The model under review builds one solid part; all positions refer to its coordinate system, in mm. A direction names the side the tool comes from. Coordinates: 2 decimals unless noted, no trailing zeros. Order: outer loops, then holes, each group sorted by start corner. A loop starts at its lowest first (then second) coordinate and runs counter-clockwise, first axis right, second up.
```python
from build123d import *

# Parameters (mm, degrees)
SKETCH1_R                = 36.8
SKETCH1_R_2              = 35.2
BOSS_EXTRUDE1_DEPTH      = 100
BOSS_EXTRUDE2_DEPTH      = 10
BOSS_EXTRUDE2_DEPTH_BACK = 5
SKETCH2_R                = 38.3
SKETCH2_R_2              = 36.8
CHAMFER1_SIZE            = 1.5
BOSS_EXTRUDE3_START      = 30
BOSS_EXTRUDE3_DEPTH      = 30
SKETCH7_R                = 1.75
CUT_EXTRUDE1_DEPTH       = 116.043019012
CUT_EXTRUDE2_REACH       = 153.112
CUT_EXTRUDE3_REACH       = 138.3
CUT_EXTRUDE3_END_RADIUS  = 35.2
SKETCH9_R                = 5


with BuildPart() as part:
    # Sketch1 → Boss-Extrude1 (new body)
    with BuildSketch(Plane.XY):
        Circle(SKETCH1_R)
        Circle(SKETCH1_R_2, mode=Mode.SUBTRACT)
    extrude(amount=BOSS_EXTRUDE1_DEPTH)

    # Sketch2 → Boss-Extrude2 (add, two sides: drawn at the far end of the back side and taken through both)
    with BuildSketch(Plane(origin=(0, 0, 0), x_dir=(-1, 0, 0), z_dir=(0, 0, -1)).offset(-BOSS_EXTRUDE2_DEPTH_BACK)):
        Circle(SKETCH2_R)
        Circle(SKETCH2_R_2, mode=Mode.SUBTRACT)
    extrude(amount=BOSS_EXTRUDE2_DEPTH + BOSS_EXTRUDE2_DEPTH_BACK)

    # Chamfer1
    chamfer1_edges = [part.edges().sort_by_distance(p)[0] for p in [
        (-36.8, 0, 5),
    ]]
    chamfer(chamfer1_edges, length=CHAMFER1_SIZE - 0.0001)  # a hair under: the kernel refuses the full size

    # Sketch6 → Boss-Extrude3 (add)
    with BuildSketch(Plane(origin=(0, 0, -10), x_dir=(-1, 0, 0), z_dir=(0, 0, -1)).offset(BOSS_EXTRUDE3_START)):
        with BuildLine():
            Line((-31.046363436, 22.427958387), (-32.43120853, 23.227499075))
            Line((-32.43120853, 23.227499075), (-35.462297443, 24.977499075))
            Line((-35.462297443, 24.977499075), (-38.147666087, 26.527897384))
            Line((-38.147666087, 26.527897384), (-39.147666087, 24.795846576))
            Line((-39.147666087, 24.795846576), (-36.462297443, 23.245448267))
            Line((-36.462297443, 23.245448267), (-33.43120853, 21.495448267))
            Line((-33.43120853, 21.495448267), (-32.177933832, 20.771869783))
            Line((-32.177933832, 20.771869783), (-30.861043972, 20.045846576))
            ThreePointArc((-30.861043972, 20.045846576), (18.4, 31.869734859), (32.790734361, -16.703524779))
            Line((32.790734361, -16.703524779), (34.077933832, -17.480973249))
            Line((34.077933832, -17.480973249), (35.33120853, -18.204551733))
            Line((35.33120853, -18.204551733), (38.362297443, -19.954551733))
            Line((38.362297443, -19.954551733), (41.047666087, -21.504950042))
            Line((41.047666087, -21.504950042), (42.047666087, -19.772899234))
            Line((42.047666087, -19.772899234), (39.362297443, -18.222500925))
            Line((39.362297443, -18.222500925), (36.33120853, -16.472500925))
            Line((36.33120853, -16.472500925), (34.946363436, -15.672960237))
            ThreePointArc((34.946363436, -15.672960237), (19.15, 33.168772965), (-31.046363436, 22.427958387))
        make_face()
        with BuildLine():
            Line((-34.946363436, 15.672960237), (-36.33120853, 16.472500925))
            Line((-36.33120853, 16.472500925), (-39.362297443, 18.222500925))
            Line((-39.362297443, 18.222500925), (-42.047666087, 19.772899234))
            Line((-42.047666087, 19.772899234), (-41.047666087, 21.504950042))
            Line((-41.047666087, 21.504950042), (-38.362297443, 19.954551733))
            Line((-38.362297443, 19.954551733), (-35.33120853, 18.204551733))
            Line((-35.33120853, 18.204551733), (-34.077933832, 17.480973249))
            Line((-34.077933832, 17.480973249), (-32.743288904, 16.796339832))
            ThreePointArc((-32.743288904, 16.796339832), (-18.4, -31.869734859), (30.917701437, -19.958350079))
            Line((30.917701437, -19.958350079), (32.177933832, -20.771869783))
            Line((32.177933832, -20.771869783), (33.43120853, -21.495448267))
            Line((33.43120853, -21.495448267), (36.462297443, -23.245448267))
            Line((36.462297443, -23.245448267), (39.147666087, -24.795846576))
            Line((39.147666087, -24.795846576), (38.147666087, -26.527897384))
            Line((38.147666087, -26.527897384), (35.462297443, -24.977499075))
            Line((35.462297443, -24.977499075), (32.43120853, -23.227499075))
            Line((32.43120853, -23.227499075), (31.046363436, -22.427958387))
            ThreePointArc((31.046363436, -22.427958387), (-19.15, -33.168772965), (-34.946363436, 15.672960237))
        make_face()
    extrude(amount=-BOSS_EXTRUDE3_DEPTH)

    # Sketch7 → Cut-Extrude1 (cut, symmetric)
    with BuildSketch(Plane(origin=(0, 0, 0), x_dir=(0, 0, 1), z_dir=(0.500000000000001, -0.866025403784438, 0))):
        with Locations(Location((-29.75, 41.45, 0), (0, 0, 270))):
            Circle(SKETCH7_R)
        with Locations(Location((-15.25, 41.45, 0), (0, 0, 270))):
            Circle(SKETCH7_R)
    cut_extrude1 = extrude(amount=CUT_EXTRUDE1_DEPTH, both=True, mode=Mode.SUBTRACT)

    # Mirror1: Cut-Extrude1 across plane
    add(cut_extrude1.mirror(Plane(origin=(0, 0, 0), x_dir=(0, 0, 1), z_dir=(0.866025403784438, 0.500000000000001, 0))), mode=Mode.SUBTRACT)

    # Cut-Extrude2: up to this face of the body (flat: up to its plane)
    cut_extrude2_end = Plane(part.part.faces().sort_by_distance((35.759138818, 0, 0))[0])
    # Sketch8 → Cut-Extrude2 (cut, up to the picked face)
    with BuildSketch(Plane(origin=(0, 0, -40), x_dir=(-1, 0, 0), z_dir=(0, 0, -1)), mode=Mode.PRIVATE) as cut_extrude2_sk1:
        with BuildLine():
            ThreePointArc((31.085732423, -20.066819373), (32.069109105, -18.454599459), (32.968944874, -16.794304805))
            ThreePointArc((32.968944874, -16.794304805), (18.5, 32.04293994), (-31.028767037, 20.154791395))
            ThreePointArc((-31.028767037, 20.154791395), (-32.016706501, 18.545363432), (-32.921241561, 16.887624287))
            ThreePointArc((-32.921241561, 16.887624287), (-18.5, -32.04293994), (31.085732423, -20.066819373))
        make_face()
    cut_extrude2_tool1 = split(extrude(cut_extrude2_sk1.sketch, amount=-CUT_EXTRUDE2_REACH, mode=Mode.PRIVATE), bisect_by=cut_extrude2_end, keep=Keep.BOTH, mode=Mode.PRIVATE)
    add(cut_extrude2_tool1.solids().sort_by(Axis((0, 0, -40), (0, 0, 1)))[0], mode=Mode.SUBTRACT)

    # Cut-Extrude3: up to this cylinder (the profile starts outside it)
    cut_extrude3_end = Plane(origin=(0, 0, 15), z_dir=(0, 0, -1)) * Cylinder(CUT_EXTRUDE3_END_RADIUS, 348, mode=Mode.PRIVATE)
    # Sketch9 → Cut-Extrude3 (cut, up to the surface)
    with BuildSketch(Plane(origin=(-18.4, 31.869734859, 0), x_dir=(0.8660254037844382, 0.500000000000001, 0), z_dir=(-0.500000000000001, 0.8660254037844382, 0)), mode=Mode.PRIVATE) as cut_extrude3_sk1:
        with Locations(Location((0, -15, 0), (0, 0, 180))):
            Circle(SKETCH9_R)
    cut_extrude3_tool1 = extrude(cut_extrude3_sk1.sketch, amount=-CUT_EXTRUDE3_REACH, mode=Mode.PRIVATE) - cut_extrude3_end
    add(cut_extrude3_tool1.solids().sort_by_distance((-18.4, 31.869735, 15))[0], mode=Mode.SUBTRACT)


solid = part.part
```
(1) Machinability: for faces 1 (the face through (-22, 31, -40)), 2 (the face through (38, 18, -10)), 3 (the face through (-38, -19, -10)), which of the approach directions +Z, -Z, +X, -X, +Y, -Y give a long, thin tool a straight path to every point of the face, cutting with its end or side? Answer none if there is none.
A:
face 1: -Z, +X, -X, +Y, -Y
face 2: +Z, +X, +Y
face 3: +Z, -X, -Y
(2) For pin 1 Ø6.5 at (x, y) = (-36, -24) entering from +Z; pin 2 Ø2.5 at (x, y) = (32, 18.5) entering from -Z; pin 3 Ø12 at (x, z) = (8.5, 30) entering from -Y (3 decimals); pin 4 Ø6 at (y, z) = (-21, -14.5) entering from -X, all flat-tipped, find the tip position at first contact; note any pin that passes through.
A:
pin 1: stops at z = -10
pin 2: stops at z = -10
pin 3: stops at y = -36.715
pin 4: stops at x = -42.05
(3) We need section C-C, the plane z = 23.5. Write out the cut boundary in (x, y).
A:
outline: circle Ø73.6 at (0, 0); hole circle Ø70.4 at (0, 0)
(4) We need section D-D, the plane y = 32. Count the separate pieces of the cut face and the enclosed holes in it, and give its area (3 significant figures).
A:
separate pieces: 3
enclosed holes: 0
area: 900 mm2
(5) Wall thickness on probe 1 along X at (y, z) = (0, -25.5); probe 2 along Y at (x, z) = (1, 82); probe 3 along Y at (x, z) = (31.5, -5): over which ranges is each line inside the solid? List them lowest first.
A:
probe 1: x = -38.3 to -37, 37 to 38.3
probe 2: y = -36.79 to -35.19, 35.19 to 36.79
probe 3: y = -21.79 to -19.41, 19.41 to 21.79
(6) Draft analysis for pull direction Z (two halves, no side actions). For faces 4 (the face through (-36.64, -17.82, -31.3)), 5 (the face through (-33, -19, -10)), 6 (the face through (35, 24, -10)), state which applies: released by +Z, released by -Z, zero draft, split by the parting line, or undercut.
A:
face 4: undercut
face 5: released by -Z
face 6: released by +Z
